Geometry: final body of the model. Coordinates: model frame, mm. Face numbers are marked on the shaded views. A direction names the side the tool comes from. Give positions to 0.01 mm unless a question says otherwise; leave off trailing zeros. Loops run counter-clockwise (first coordinate to the right, second up) from the corner with the lowest first, then second, coordinate; pieces in that order, holes last. Notation, with made-up numbers: (49, 15.5) - (76, 15.5) arc R4 cw to (76, 21.5) - close; hole circle Ø1 at (13, 50). An arc over 180 degrees is marked (long way). Answer in a Markdown table with one row per item.
from build123d import *

# Parameters (mm, degrees)
REDONDEO1_R = 1


with BuildPart() as part:
    # Croquis1 → Revolución1 (revolve)
    with BuildSketch(Plane.XY):
        Polygon((0, 7), (0, -7), (0, -10), (0, -68.645053037), (-1.35, -68.645053037), (-1.35, -56.645053037), (-0.8, -56.645053037), (-0.8, -18.645053037), (-2.5, -18.645053037), (-2.5, -9.645053037), (-3.5, -7), (-3.5, 7), (-2.5, 9.645053037), (-2.5, 18.645053037), (-0.8, 18.645053037), (-0.8, 56.645053037), (-1.35, 56.645053037), (-1.35, 68.645053037), (0, 68.645053037), (0, 10), align=None)
    revolve(axis=Axis((0, 68.645053037, 0), (0, -1, 0)))

    # Croquis2 → Revolución2 (revolve)
    with BuildSketch(Plane.XY):
        Polygon((0, 0), (0, 3.5), (-12, 2.5), (-12, 0), align=None)
    revolve(axis=Axis((0, 0, 0), (-1, 0, 0)))

    # Redondeo1
    redondeo1_edges = [part.edges().sort_by_distance(p)[0] for p in [
        (1.35, -68.645053037, 0),
        (1.35, 68.645053037, 0),
    ]]
    fillet(redondeo1_edges, radius=REDONDEO1_R)


solid = part.part
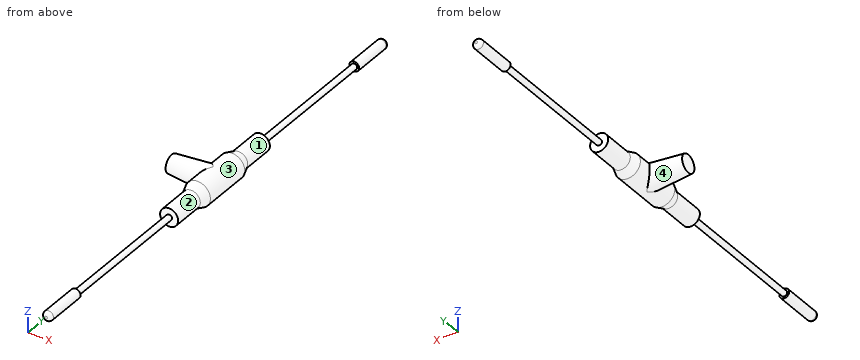
Q1. Reachability of the marked faces 1 and 2 from +Z, -Z, +X, -X, +Y, -Y: full face, straight path, thin tool, end or side. Return the list, or none.
Check values:
| item | result |
|---|---|
| face 1 | +Y |
| face 2 | -Y |
Q2. Cut plane A-A (y = -49). Output: boundary loops of the cut face in (x, z), and give its area (3 significant figures).
Check values:
| item | result |
|---|---|
| outline | circle Ø1.6 at (0, 0) |
| area | 2.01 mm² |
Q3. First-contact query: pin 1 (3 mm diameter, centred on x = -2, y = 44.5, fed in from +Z); pin 2 (1 mm diameter, centred on x = -3, y = 7.5, fed in from -Z); pin 3 (1 mm diameter, centred on x = -6.5, z = 1, fed in from +Y); pin 4 (3 mm diameter, centred on x = -4, y = -20.5, fed in from +Z) (3 decimals). Flat tips, straight axial feed; report the tip coordinate or a pass-through.
Check values:
| item | result |
|---|---|
| pin 1 | z = 0.62 |
| pin 2 | z = -2.24 |
| pin 3 | y = 2.93 |
| pin 4 | through |
Q4. Draft query along X for the marked faces 3 and 4. Return one class per face: pulls with the +X half, pulls with the -X half, needs draft (parallel to the pull), parting line crosses it, or undercut.
Check values:
| item | result |
|---|---|
| face 3 | parting line crosses it |
| face 4 | pulls with the -X half |
Q5. Cut plane B-B (x = -8.75). Output: boundary loops of the cut face in (y, z).
Check values:
| item | result |
|---|---|
| outline | circle Ø5.54 at (0, 0) |
Q6. Material intervals for line 1 along Y through (x, z) = (-10.5, -2.25); line 2 along X through (y, z) = (34, 0); line 3 along Y through (x, z) = (0.25, 2.25), sorted ascending.
Check values:
| item | result |
|---|---|
| line 1 | -1.35 to 1.35 |
| line 2 | -0.8 to 0.8 |
| line 3 | -18.65 to 18.65 |
Q7. Cut plane C-C (y = 0). Output: boundary loops of the cut face in (x, z), and give its area (3 significant figures).
Check values:
| item | result |
|---|---|
| outline | (-12, -2.5) - (-0.58, -3.45) arc R3.5 ccw (long way) to (-0.58, 3.45) - (-12, 2.5) - close |
| area | 91.3 mm² |
